from build123d import *

# Parameters (mm, degrees)
F1_DEPTH = 12
F3_DEPTH = 2
F4_SIZE2 = 11.99999
F4_SIZE  = 2.550669
F5_R     = 3


# Not quite as in the source:
# - a fillet or chamfer is up to 0.001 mm smaller than in the source, because OpenCascade refuses the exact size


with BuildPart() as f1:
    # F0 (on Top) → F1 (new body)
    with BuildSketch(Plane.XY):
        with BuildLine():
            Line((15.6635716436, 55.8448970217), (0, 30.6775543541))
            Line((0, 30.6775543541), (-15.6635716436, 55.8448970217))
            ThreePointArc((-15.6635716436, 55.8448970217), (-50.2294734195, 29), (-56.1948853143, -14.3573975535))
            Line((-56.1948853143, -14.3573975535), (-26.5675413967, -15.3387771771))
            Line((-26.5675413967, -15.3387771771), (-40.5313136707, -41.4874994682))
            ThreePointArc((-40.5313136707, -41.4874994682), (0, -58), (40.5313136707, -41.4874994682))
            Line((40.5313136707, -41.4874994682), (26.5675413967, -15.3387771771))
            Line((26.5675413967, -15.3387771771), (56.1948853143, -14.3573975535))
            ThreePointArc((56.1948853143, -14.3573975535), (50.2294734195, 29), (15.6635716436, 55.8448970217))
        make_face()
        with BuildLine():
            ThreePointArc((-53.7981180404, -11.435142995), (-47.6313972081, 27.5), (-16.9959346906, 52.3081083962))
            Line((-16.9959346906, 52.3081083962), (0, 25))
            Line((0, 25), (16.9959346906, 52.3081083962))
            ThreePointArc((16.9959346906, 52.3081083962), (47.6313972081, 27.5), (53.7981180404, -11.435142995))
            Line((53.7981180404, -11.435142995), (21.6506350946, -12.5))
            Line((21.6506350946, -12.5), (36.8021833497, -40.8729654013))
            ThreePointArc((36.8021833497, -40.8729654013), (0, -55), (-36.8021833497, -40.8729654013))
            Line((-36.8021833497, -40.8729654013), (-21.6506350946, -12.5))
            Line((-21.6506350946, -12.5), (-53.7981180404, -11.435142995))
        make_face(mode=Mode.SUBTRACT)
    extrude(amount=F1_DEPTH)

    # F2 (on face) → F3 (join)
    with BuildSketch(Plane(origin=(0, 0, 0), x_dir=(1, 0, 0), z_dir=(0, 0, -1))):
        with BuildLine():
            Line((31.4844476987, 18.1775543541), (44.2174856505, 42.0215892459))
            ThreePointArc((44.2174856505, 42.0215892459), (0, 61), (-44.2174856505, 42.0215892459))
            Line((-44.2174856505, 42.0215892459), (-31.4844476987, 18.1775543541))
            Line((-31.4844476987, 18.1775543541), (-58.5005066196, 17.2826712419))
            ThreePointArc((-58.5005066196, 17.2826712419), (-52.8275496309, -30.5), (-14.2830209691, -59.3042604877))
            Line((-14.2830209691, -59.3042604877), (0, -36.3551087083))
            Line((0, -36.3551087083), (14.2830209691, -59.3042604877))
            ThreePointArc((14.2830209691, -59.3042604877), (52.8275496309, -30.5), (58.5005066196, 17.2826712419))
            Line((58.5005066196, 17.2826712419), (31.4844476987, 18.1775543541))
        make_face()
        with BuildLine():
            Line((-21.6506350946, 12.5), (-36.8021833497, 40.8729654013))
            ThreePointArc((-36.8021833497, 40.8729654013), (0, 55), (36.8021833497, 40.8729654013))
            Line((36.8021833497, 40.8729654013), (21.6506350946, 12.5))
            Line((21.6506350946, 12.5), (53.7981180404, 11.435142995))
            ThreePointArc((53.7981180404, 11.435142995), (47.6313972081, -27.5), (16.9959346906, -52.3081083962))
            Line((16.9959346906, -52.3081083962), (0, -25))
            Line((0, -25), (-16.9959346906, -52.3081083962))
            ThreePointArc((-16.9959346906, -52.3081083962), (-47.6313972081, -27.5), (-53.7981180404, 11.435142995))
            Line((-53.7981180404, 11.435142995), (-21.6506350946, 12.5))
        make_face(mode=Mode.SUBTRACT)
    extrude(amount=F3_DEPTH)

    # F4 (size 2.55067874 and 12 in the source; OpenCascade refuses exactly that, so slightly less here)
    f4_edges = [f1.edges().sort_by_distance(p)[0] for p in [
        (-41.381213, -14.848087, 12),
        (-33.549428, -28.413138, 12),
        (0, -58, 12),
        (-50.229473, 29, 12),
        (-7.831786, 43.261226, 12),
        (7.831786, 43.261226, 12),
        (50.229473, 29, 12),
        (41.381213, -14.848087, 12),
        (33.549428, -28.413138, 12),
    ]]
    f4_side = f1.faces().sort_by_distance((0, -56.37468, 12))[0]
    chamfer(f4_edges, length=F4_SIZE, length2=F4_SIZE2, reference=f4_side)

    # F5
    f5_edges = [f1.edges().sort_by_distance(p)[0] for p in [
        (-58.500507, -17.282671, -1),
        (-31.484448, -18.177554, -1),
        (-44.217486, -42.021589, -1),
        (44.217486, -42.021589, -1),
        (31.484448, -18.177554, -1),
        (58.500507, -17.282671, -1),
        (14.283021, 59.30426, -1),
        (0, 36.355109, -1),
        (-14.283021, 59.30426, -1),
    ]]
    fillet(f5_edges, radius=F5_R)


solid = f1.part
Source: CAD feature listing. Evaluate the final solid. Frame: model axes, mm. A direction names the side the tool comes from. Give positions to 0.01 mm unless a question says otherwise; leave off trailing zeros. Loops run counter-clockwise (first coordinate to the right, second up) from the corner with the lowest first, then second, coordinate; pieces in that order, holes last. Notation, with made-up numbers: (89.25, -34.75) -> (94.25, -34.75) arc R10 cw to (94.25, -16.75) -> close; hole circle Ø6 at (76.5, 31.5). An arc over 180 degrees is marked (long way). Use a Markdown table: item, result. Add a question column.
1) Line query: line 1 along X through (y, z) = (30, -1); line 2 along Y through (x, z) = (36.5, 6.75); line 3 along X through (y, z) = (34, 6.75). Output: solid intervals per line, ascending. Write a range as [from, to].
2) First-contact query: pin 1 (2 mm diameter, centred on x = -35, z = 5, fed in from +Y); pin 2 (1.5 mm diameter, centred on y = 30, z = 4.5, fed in from -X); pin 3 (3 mm diameter, centred on y = -30, z = 1, fed in from -X). Flat tips, straight axial feed; report the tip coordinate or a pass-through.
3) Section query A-A, the plane z = 9.5. Return the cut outline in (x, y), then the cut area to 3 significant figures.
4) Reachability of faces 1 (the face through (-0.564, -54.997, 5.098)), 2 (the face through (-7.906, 49.058, -0.986)), 3 (the face through (-31.364, -26.99, 5.916)) from +Z, -Z, +X, -X, +Y, -Y: full face, straight path, thin tool, end or side. Return the list, or none.
5) Section query C-C, the plane y = 35. Count the separate pieces of the cut face and the enclosed holes in it, then the cut area to 3 significant figures.
6) Pull-direction query (Y, two-part tool) for faces 4 (the face through (52.494, 31.07, -0.986)), 5 (the face through (-8.4, 38.5, 5.1)), 6 (the face through (-7.692, 40.657, 5.916)); classes: +Y half, -Y half, draft (parallel to the pull), parting line (faces both ways), or undercut.
Numbers:
| question | item | result |
|---|---|---|
| 1 | line 1 | x = [-53.11, -46.1], [-3.11, 3.11], [46.1, 53.11] |
| 1 | line 2 | y = [-43.21, -41.14], [-40.31, -36.98], [-13.57, -12.01], [41.14, 43.21] |
| 1 | line 3 | x = [-45.21, -43.23], [-5.6, -3.76], [3.76, 5.6], [43.23, 45.21] |
| 2 | pin 1 | stops at y = 45.72 |
| 2 | pin 2 | stops at x = -49.01 |
| 2 | pin 3 | stops at x = -38.39 |
| 3 | outline | (-54.59, -12.39) -> (-23.26, -13.43) -> (-38.03, -41.08) arc R55.98 ccw to (38.03, -41.08) -> (23.26, -13.43) -> (54.59, -12.39) arc R55.98 ccw to (16.57, 53.47) -> (0, 26.86) -> (-16.57, 53.47) arc R55.98 ccw to start; hole (-53.8, -11.44) -> (-21.65, -12.5) -> (-36.8, -40.87) arc R55 ccw to (36.8, -40.87) -> (21.65, -12.5) -> (53.8, -11.44) arc R55 ccw to (17, 52.31) -> (0, 25) -> (-17, 52.31) arc R55 ccw to start |
| 3 | area | 428 mm2 |
| 4 | face 1 | +Z, -Z |
| 4 | face 2 | +Z, -Z, +Y |
| 4 | face 3 | +Z, -X |
| 5 | separate pieces | 3 |
| 5 | enclosed holes | 0 |
| 5 | area | 157 mm2 |
| 6 | face 4 | parting line |
| 6 | face 5 | undercut |
| 6 | face 6 | +Y half |
